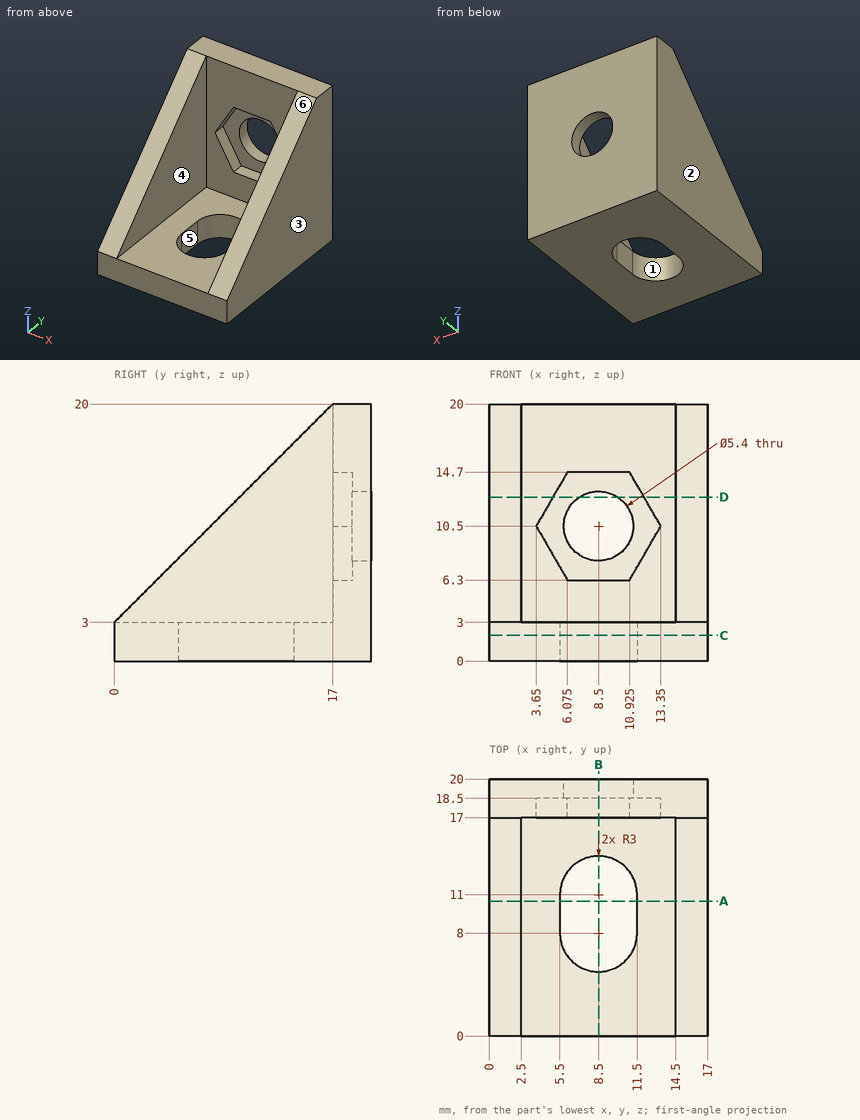
Here's the drawing with two shaded views (mm, measured from the low corner). I have some questions. A direction names the side the tool comes from. Give positions to 0.01 mm unless a question says otherwise; leave off trailing zeros. Loops run counter-clockwise (first coordinate to the right, second up) from the corner with the lowest first, then second, coordinate; pieces in that order, holes last. Notation, with made-up numbers: (-36.5, 31.25) - (-15.5, 31.25) arc R4 cw to (-15.5, 36.25) - close; hole circle Ø3 at (-39.75, 83). An arc over 180 degrees is marked (long way). Return JSON: item names as keys, results as strings.
1. I'm going to push flat-ended pins straight in: pin 1 Ø4 at (x, z) = (10.5, 10) entering from -Y; pin 2 Ø5 at (x, y) = (8, 2.5) entering from +Z; pin 3 Ø5 at (x, y) = (3, 12) entering from +Z. Where does each tip first touch, or does it pass through?
Output values:
{"pin 1": "stops at y = 18.5", "pin 2": "stops at z = 3", "pin 3": "stops at z = 17.45"}
2. We'd pull the mould along X, two halves only. Please class the marked faces 1, 2 and 3: +X half, -X half, draft (parallel to the pull), parting line (faces both ways), or undercut.
Output values:
{"face 1": "undercut", "face 2": "-X half", "face 3": "+X half"}
3. I want a section at D-D on z = 12.75. Please give me the cut outline in (x, y).
Output values:
{"outline": "(0, 9.75) - (2.5, 9.75) - (2.5, 17) - (4.95, 17) - (4.95, 18.5) - (7.01, 18.5) - (7.01, 20) - (0, 20) - close; (9.99, 18.5) - (12.05, 18.5) - (12.05, 17) - (14.5, 17) - (14.5, 9.75) - (17, 9.75) - (17, 20) - (9.99, 20) - close"}
4. If I drill on line 1 (Z direction, x = 8.5, y = 19.3); line 2 (X direction, y = 18.9, z = 10.5); line 3 (Z direction, x = 13.5, y = 15.5), over which ranges is the centre line in solid material (lowest first)?
Output values:
{"line 1": "z = 0 to 7.8, 13.2 to 20", "line 2": "x = 0 to 5.8, 11.2 to 17", "line 3": "z = 0 to 3"}
5. I want a section at B-B on x = 8.5. Please give me the cut outline in (y, z).
Output values:
{"outline": "(0, 0) - (5, 0) - (5, 3) - (0, 3) - close; (14, 0) - (20, 0) - (20, 7.8) - (18.5, 7.8) - (18.5, 6.3) - (17, 6.3) - (17, 3) - (14, 3) - close; (17, 14.7) - (18.5, 14.7) - (18.5, 13.2) - (20, 13.2) - (20, 20) - (17, 20) - close"}
6. I want a section at C-C on z = 2. Please give me the cut outline in (x, y).
Output values:
{"outline": "(0, 0) - (17, 0) - (17, 20) - (0, 20) - close; hole (5.5, 8) arc R3 ccw to (11.5, 8) - (11.5, 11) arc R3 ccw to (5.5, 11) - close"}
7. For the marked faces 4, 5 and 6, which set-ups out of +Z, -Z, +X, -X, +Y, -Y let a thin tool reach every point of the face, with its end or its side?
Output values:
{"face 4": "+Z, -Y", "face 5": "+Z, -Z", "face 6": "+Z, +X, -X, -Y"}
8. I want a section at A-A on y = 10.5. Please give me the cut outline in (x, z), and give its area (3 significant figures).
Output values:
{"outline": "(0, 0) - (5.5, 0) - (5.5, 3) - (2.5, 3) - (2.5, 13.5) - (0, 13.5) - close; (11.5, 0) - (17, 0) - (17, 13.5) - (14.5, 13.5) - (14.5, 3) - (11.5, 3) - close", "area": "85.5 mm²"}
